```python
from build123d import *

# Parameters (mm, degrees)
BOSS_EXTRUDE1_DEPTH     = 3
SKETCH2_R               = 12
SKETCH2_R_2             = 11
SKETCH2_W               = 3
SKETCH2_H               = 14.132174157
CUT_EXTRUDE1_DEPTH      = 1
CUT_EXTRUDE1_DEPTH_BACK = 4
CUT_EXTRUDE2_DEPTH      = 10


with BuildPart() as part:
    # Sketch1 → Boss-Extrude1 (new body)
    with BuildSketch(Plane.XY):
        Polygon((-415, 0), (-415, 30), (-405, 30), (-405, 32.5), (-0.255808808, 54.019626957), (0, 28.020885413), (-405, 0), align=None)
    extrude(amount=BOSS_EXTRUDE1_DEPTH)

    # Sketch2 → Cut-Extrude1 (cut, two sides)
    with BuildSketch(Plane.XY.offset(3)) as cut_extrude1_sk:
        with Locations((-368.509952953, 17.345136607)):
            Circle(SKETCH2_R)
        with Locations((-340.019905905, 19.176130471)):
            Circle(SKETCH2_R)
        with Locations((-311.529858858, 21.007124335)):
            Circle(SKETCH2_R)
        with Locations((-283.039811811, 22.8381182)):
            Circle(SKETCH2_R)
        with Locations((-254.549764764, 24.669112064)):
            Circle(SKETCH2_R)
        with Locations((-190, 28.817586197)):
            Circle(SKETCH2_R_2)
        with Locations((-161.439118955, 30.65313241)):
            Circle(SKETCH2_R_2)
        with Locations((-132.878237911, 32.488678622)):
            Circle(SKETCH2_R_2)
        with Locations((-104.317356866, 34.324224835)):
            Circle(SKETCH2_R_2)
        with Locations((-75.756475821, 36.159771047)):
            Circle(SKETCH2_R_2)
        with Locations((-47.195594776, 37.99531726)):
            Circle(SKETCH2_R_2)
        with Locations((-18.634713732, 39.830863473)):
            Circle(SKETCH2_R_2)
        with Locations((-226.059717716, 26.500105928)):
            Circle(SKETCH2_R)
        with Locations((-207.5, 20.626811871)):
            Rectangle(SKETCH2_W, SKETCH2_H)
    extrude(amount=CUT_EXTRUDE1_DEPTH, mode=Mode.SUBTRACT)
    extrude(cut_extrude1_sk.sketch, amount=-CUT_EXTRUDE1_DEPTH_BACK, mode=Mode.SUBTRACT)

    # Sketch3 → Cut-Extrude2 (cut)
    with BuildSketch(Plane.XY.offset(3)):
        Polygon((-0.255808808, 54.019626957), (-3.196773149, 53.8632604), (-3.196773149, 48.019626957), (-0.196773149, 48.019626957), align=None)
        Polygon((0, 28.020885413), (-3.059035659, 27.809238777), (-3.059035659, 34.020885413), (-0.059035659, 34.020885413), align=None)
    extrude(amount=-CUT_EXTRUDE2_DEPTH, mode=Mode.SUBTRACT)


solid = part.part
```
Work out the finished part from the listing and answer in its coordinate system (mm). Coordinates: 2 decimals unless noted, no trailing zeros. Loops run counter-clockwise (first coordinate to the right, second up) from the corner with the lowest first, then second, coordinate; pieces in that order, holes last. Notation, with made-up numbers: M 38.5,86.25 L 53.5,86.25 A27 cw 53.5,121.25 Z; hole C -30.5,-19 d5. An arc over 180 degrees is marked long. Use CSV: the item, a comma, the result in double quotes. Start each with the question number.
(1) Given pin 1 Ø0.9 at (y, z) = (51.5, 1.5) entering from +X; pin 2 Ø17.5 at (x, y) = (-161.44, 30.65) entering from +Z; pin 3 Ø1.5 at (x, z) = (-290.5, 1) entering from +Y; pin 4 Ø1.5 at (x, z) = (-128.5, 1.5) entering from +Y, each flat-ended and moving along its own axis, determine where each tip first touches the part or whether it passes through.
(2) Find section C-C, the plane x = -220.5. Give the vertices of the cut face in (y, z), then the cut area to 3 significant figures.
(3) Consider line 1 (Y direction, x = -252, z = 0.2); line 2 (Y direction, x = -373.5, z = 0.95); line 3 (Y direction, x = -205, z = 2.9). Determine where each line is inside the solid, lowest interval first.
(4) Find section B-B, the plane z = 1.55. State how many separate pieces and enclosed holes the cut face has, then the cut area to 3 significant figures.
(5) For a pull along Y with two mould halves and no side action, classify faces 1 (the face through (-143.868, 32.972, 1.521)), 2 (the face through (-305.628, 6.875, 1.479)), 3 (the face through (-206.911, 43.032, 1.479)) as +Y half, -Y half, draft (parallel to the pull), parting line (faces both ways), or undercut.
(6) Find section A-A, the plane x = -129. Give the vertices of the cut face in (y, z).
Recorded:
1,pin 1,"stops at x = -3.2"
1,pin 2,"passes through"
1,pin 3,"stops at y = 38.63"
1,pin 4,"stops at y = 47.24"
2,outline,"M 12.77,0 L 15.87,0 L 15.87,3 L 12.77,3 Z; M 37.13,0 L 42.31,0 L 42.31,3 L 37.13,3 Z"
2,area,"24.8 mm^2"
3,line 1,"y = 10.59 to 12.94, 36.4 to 40.63"
3,line 2,"y = 2.18 to 6.43, 28.26 to 34.17"
3,line 3,"y = 13.84 to 43.13"
4,separate pieces,"1"
4,enclosed holes,"13"
4,area,"6,690 mm^2"
5,face 1,"undercut"
5,face 2,"-Y half"
5,face 3,"+Y half"
6,outline,"M 19.1,0 L 22.2,0 L 22.2,3 L 19.1,3 Z; M 42.78,0 L 47.17,0 L 47.17,3 L 42.78,3 Z"
